Build history of the part. All positions in model axes, mm. A direction names the side the tool comes from. Round coordinates to 2 decimals unless told otherwise and drop trailing zeros. Order: outer loops, then holes, each group sorted by start corner. A loop starts at its lowest first (then second) coordinate and runs counter-clockwise, first axis right, second up. Notation, with made-up numbers: (53, 46.5) -> (107, 46.5) arc R27 cw to (107, 64.5) -> close; hole circle Ø8 at (-29, 89). An arc over 180 degrees is marked (long way). Use a Markdown table: item, result. Add a question column.
Item 1: Probe L1, parallel to X at y = 33.5, z = 6; L2, parallel to Y at x = 12.75, z = 4.25; L3, parallel to Y at x = -36, z = 8.5. List the from-to ranges inside material, lowest first.
Item 2: 3-axis set-ups, long thin cutter, end or side, ignore diameter. For faces 4 (the face through (35, 147, 5)), 5 (the face through (-1, 76, 10)): which of +Z, -Z, +X, -X, +Y, -Y reach the whole face in a straight line?
Item 3: Two-plate mould, pull along Y, no slides. Class faces 1 (the face through (-1, 0, 5)), 2 (the face through (-45, 74, 5)), 3 (the face through (-35, 43, 5)): released by +Y, released by -Y, zero draft, split by the parting line, or undercut.
Item 4: Slice it at D-D, the plane x = -12.75. Give the cut face in (y, z).
Item 5: Slice it at C-C, the plane z = 1.75. State how many separate pieces and enclosed holes the cut face has, plus the area to 3 significant figures.
Item 6: Slice it at A-A, the plane y = 87.75. Give the cut face in (x, z), plus the area to 3 significant figures.
Item 7: Slice it at B-B, the plane x = -35. Give the cut face in (y, z).
from build123d import *

# Parameters (mm, degrees)
SKETCH_2_W          = 90
SKETCH_2_H          = 150
EXTRUDE_1_DEPTH     = 10
SKETCH_3_W          = 57.822110836
SKETCH_3_H          = 142.808753936
EXTRUDE_2_DEPTH     = 10
CUT_EXTRUDE_1_REACH = 12
SKETCH_10_R         = 3.4


with BuildPart() as part:
    # 草圖2 → 填料-伸長1 (new body)
    with BuildSketch(Plane.XY):
        with Locations((0, 75)):
            Rectangle(SKETCH_2_W, SKETCH_2_H)
        with BuildLine():
            Line((40, 142), (40, 112))
            ThreePointArc((40, 112), (35, 107), (30, 112))
            Line((30, 112), (30, 142))
            ThreePointArc((30, 142), (35, 147), (40, 142))
        make_face(mode=Mode.SUBTRACT)
        with BuildLine():
            Line((27, 139.5), (27, 114.5))
            ThreePointArc((27, 114.5), (23.75, 111.25), (20.5, 114.5))
            Line((20.5, 114.5), (20.5, 139.5))
            ThreePointArc((20.5, 139.5), (23.75, 142.75), (27, 139.5))
        make_face(mode=Mode.SUBTRACT)
        with BuildLine():
            Line((-40, 142), (-40, 112))
            ThreePointArc((-40, 112), (-35, 107), (-30, 112))
            Line((-30, 112), (-30, 142))
            ThreePointArc((-30, 142), (-35, 147), (-40, 142))
        make_face(mode=Mode.SUBTRACT)
        with BuildLine():
            Line((-27, 139.5), (-27, 114.5))
            ThreePointArc((-27, 114.5), (-23.75, 111.25), (-20.5, 114.5))
            Line((-20.5, 114.5), (-20.5, 139.5))
            ThreePointArc((-20.5, 139.5), (-23.75, 142.75), (-27, 139.5))
        make_face(mode=Mode.SUBTRACT)
        with BuildLine():
            Line((40, 60), (40, 90))
            ThreePointArc((40, 90), (35, 95), (30, 90))
            Line((30, 90), (30, 60))
            ThreePointArc((30, 60), (35, 55), (40, 60))
        make_face(mode=Mode.SUBTRACT)
        with BuildLine():
            Line((27, 62.5), (27, 87.5))
            ThreePointArc((27, 87.5), (23.75, 90.75), (20.5, 87.5))
            Line((20.5, 87.5), (20.5, 62.5))
            ThreePointArc((20.5, 62.5), (23.75, 59.25), (27, 62.5))
        make_face(mode=Mode.SUBTRACT)
        with BuildLine():
            Line((-40, 60), (-40, 90))
            ThreePointArc((-40, 90), (-35, 95), (-30, 90))
            Line((-30, 90), (-30, 60))
            ThreePointArc((-30, 60), (-35, 55), (-40, 60))
        make_face(mode=Mode.SUBTRACT)
        with BuildLine():
            Line((-27, 62.5), (-27, 87.5))
            ThreePointArc((-27, 87.5), (-23.75, 90.75), (-20.5, 87.5))
            Line((-20.5, 87.5), (-20.5, 62.5))
            ThreePointArc((-20.5, 62.5), (-23.75, 59.25), (-27, 62.5))
        make_face(mode=Mode.SUBTRACT)
        with BuildLine():
            Line((-40, 8), (-40, 38))
            ThreePointArc((-40, 38), (-35, 43), (-30, 38))
            Line((-30, 38), (-30, 8))
            ThreePointArc((-30, 8), (-35, 3), (-40, 8))
        make_face(mode=Mode.SUBTRACT)
        with BuildLine():
            Line((-27, 10.5), (-27, 35.5))
            ThreePointArc((-27, 35.5), (-23.75, 38.75), (-20.5, 35.5))
            Line((-20.5, 35.5), (-20.5, 10.5))
            ThreePointArc((-20.5, 10.5), (-23.75, 7.25), (-27, 10.5))
        make_face(mode=Mode.SUBTRACT)
        with BuildLine():
            Line((40, 8), (40, 38))
            ThreePointArc((40, 38), (35, 43), (30, 38))
            Line((30, 38), (30, 8))
            ThreePointArc((30, 8), (35, 3), (40, 8))
        make_face(mode=Mode.SUBTRACT)
        with BuildLine():
            Line((27, 10.5), (27, 35.5))
            ThreePointArc((27, 35.5), (23.75, 38.75), (20.5, 35.5))
            Line((20.5, 35.5), (20.5, 10.5))
            ThreePointArc((20.5, 10.5), (23.75, 7.25), (27, 10.5))
        make_face(mode=Mode.SUBTRACT)
    extrude(amount=EXTRUDE_1_DEPTH)

    # 草圖3 → 填料-伸長2 (add)
    with BuildSketch(Plane.XY.offset(10)):
        with Locations((-0.145737049, 74.293544629)):
            Rectangle(SKETCH_3_W, SKETCH_3_H)
    extrude(amount=-EXTRUDE_2_DEPTH)

    # 草圖10 → 除料-伸長1 (cut, up to next)
    with BuildSketch(Plane.XY.offset(10), mode=Mode.PRIVATE) as cut_extrude_1_sk1:
        with Locations((12.75, 62.25)):
            Circle(SKETCH_10_R)
    cut_extrude_1_tool1 = extrude(cut_extrude_1_sk1.sketch, amount=-CUT_EXTRUDE_1_REACH, mode=Mode.PRIVATE) & part.part
    add(cut_extrude_1_tool1.solids().sort_by_distance((12.75, 62.25, 10))[0], mode=Mode.SUBTRACT)
    # 草圖10 → 除料-伸長1 (cut, up to next)
    with BuildSketch(Plane.XY.offset(10), mode=Mode.PRIVATE) as cut_extrude_1_sk2:
        with Locations((-12.75, 62.25)):
            Circle(SKETCH_10_R)
    cut_extrude_1_tool2 = extrude(cut_extrude_1_sk2.sketch, amount=-CUT_EXTRUDE_1_REACH, mode=Mode.PRIVATE) & part.part
    add(cut_extrude_1_tool2.solids().sort_by_distance((-12.75, 62.25, 10))[0], mode=Mode.SUBTRACT)
    # 草圖10 → 除料-伸長1 (cut, up to next)
    with BuildSketch(Plane.XY.offset(10), mode=Mode.PRIVATE) as cut_extrude_1_sk3:
        with Locations((12.75, 87.75)):
            Circle(SKETCH_10_R)
    cut_extrude_1_tool3 = extrude(cut_extrude_1_sk3.sketch, amount=-CUT_EXTRUDE_1_REACH, mode=Mode.PRIVATE) & part.part
    add(cut_extrude_1_tool3.solids().sort_by_distance((12.75, 87.75, 10))[0], mode=Mode.SUBTRACT)
    # 草圖10 → 除料-伸長1 (cut, up to next)
    with BuildSketch(Plane.XY.offset(10), mode=Mode.PRIVATE) as cut_extrude_1_sk4:
        with Locations((-12.75, 87.75)):
            Circle(SKETCH_10_R)
    cut_extrude_1_tool4 = extrude(cut_extrude_1_sk4.sketch, amount=-CUT_EXTRUDE_1_REACH, mode=Mode.PRIVATE) & part.part
    add(cut_extrude_1_tool4.solids().sort_by_distance((-12.75, 87.75, 10))[0], mode=Mode.SUBTRACT)


solid = part.part
Check sheet entries:
| question | item | result |
|---|---|---|
| 1 | L1 | -45 to -40, -30 to 30, 40 to 45 |
| 1 | L2 | 0 to 58.85, 65.65 to 84.35, 91.15 to 150 |
| 1 | L3 | 0 to 3.1, 42.9 to 55.1, 94.9 to 107.1, 146.9 to 150 |
| 2 | face 4 | +Z, -Z |
| 2 | face 5 | +Z, +X, -X, +Y, -Y |
| 3 | face 1 | released by -Y |
| 3 | face 2 | zero draft |
| 3 | face 3 | undercut |
| 4 | outline | (0, 0) -> (58.85, 0) -> (58.85, 10) -> (0, 10) -> close; (65.65, 0) -> (84.35, 0) -> (84.35, 10) -> (65.65, 10) -> close; (91.15, 0) -> (150, 0) -> (150, 10) -> (91.15, 10) -> close |
| 5 | separate pieces | 1 |
| 5 | enclosed holes | 10 |
| 5 | area | 11,100 mm2 |
| 6 | outline | (-45, 0) -> (-40, 0) -> (-40, 10) -> (-45, 10) -> close; (-30, 0) -> (-16.15, 0) -> (-16.15, 10) -> (-30, 10) -> close; (-9.35, 0) -> (9.35, 0) -> (9.35, 10) -> (-9.35, 10) -> close; (16.15, 0) -> (30, 0) -> (30, 10) -> (16.15, 10) -> close; (40, 0) -> (45, 0) -> (45, 10) -> (40, 10) -> close |
| 6 | area | 564 mm2 |
| 7 | outline | (0, 0) -> (3, 0) -> (3, 10) -> (0, 10) -> close; (43, 0) -> (55, 0) -> (55, 10) -> (43, 10) -> close; (95, 0) -> (107, 0) -> (107, 10) -> (95, 10) -> close; (147, 0) -> (150, 0) -> (150, 10) -> (147, 10) -> close |
